Source: three-view drawing plus pictorial views. Frame: mm from the lowest corner of the part. A direction names the side the tool comes from. Round coordinates to 2 decimals unless told otherwise and drop trailing zeros. Loops run counter-clockwise (first coordinate to the right, second up) from the corner with the lowest first, then second, coordinate; pieces in that order, holes last. Notation, with made-up numbers: (57.25, -4) -> (110.25, -4) arc R25 ccw to (110.25, 23) -> close; hole circle Ø1 at (63, 25). An arc over 180 degrees is marked (long way). Answer in a Markdown table with one row per item.
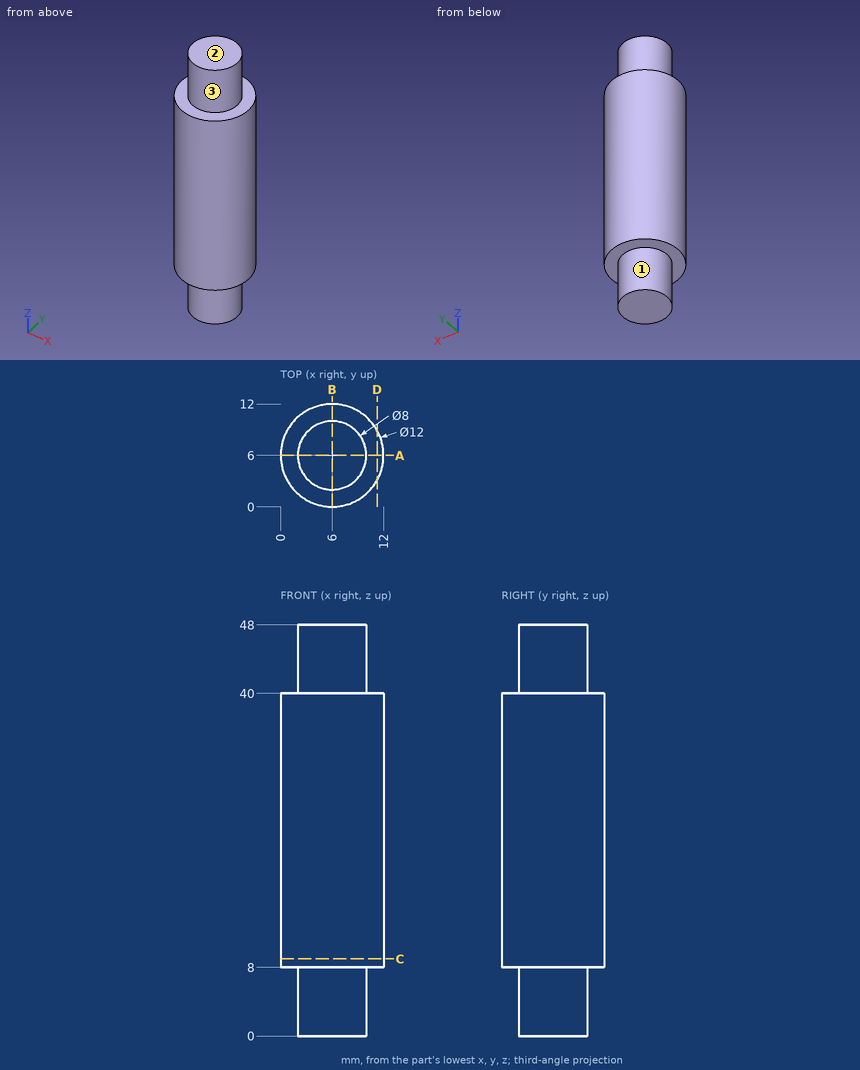
Item 1: Reachability of the marked faces 1, 2 and 3 from +Z, -Z, +X, -X, +Y, -Y: full face, straight path, thin tool, end or side. Return the list, or none.
Answer:
| item | result |
|---|---|
| face 1 | -Z |
| face 2 | +Z, +X, -X, +Y, -Y |
| face 3 | +Z |
Item 2: Cut plane D-D (x = 11.25). Output: boundary loops of the cut face in (y, z).
Answer:
| item | result |
|---|---|
| outline | (3.1, 8) -> (8.9, 8) -> (8.9, 40) -> (3.1, 40) -> close |
Item 3: Cut plane A-A (y = 6). Output: boundary loops of the cut face in (x, z), then the cut area to 3 significant figures.
Answer:
| item | result |
|---|---|
| outline | (0, 8) -> (2, 8) -> (2, 0) -> (10, 0) -> (10, 8) -> (12, 8) -> (12, 40) -> (10, 40) -> (10, 48) -> (2, 48) -> (2, 40) -> (0, 40) -> close |
| area | 512 mm² |
Item 4: Line query: probe 1 along Z at (x, y) = (9.5, 1.25); probe 2 along X at (y, z) = (6.75, 30); probe 3 along Y at (x, z) = (10, 36). Output: solid intervals per line, ascending. Write a range as [from, to].
Answer:
| item | result |
|---|---|
| probe 1 | z = [8, 40] |
| probe 2 | x = [0.05, 11.95] |
| probe 3 | y = [1.53, 10.47] |
Item 5: Cut plane C-C (z = 9). Output: boundary loops of the cut face in (x, y), then the cut area to 3 significant figures.
Answer:
| item | result |
|---|---|
| outline | circle Ø12 at (6, 6) |
| area | 113 mm² |
Item 6: Pin query (flat end, axial travel): pin 1 Ø6 at (x, y) = (6.5, 5.5) entering from -Z; pin 2 Ø1 at (x, z) = (8.5, 8.5) entering from +Y; pin 3 Ø1.5 at (y, z) = (5.5, 42.5) entering from -X; pin 4 Ø1.5 at (x, z) = (3.5, 37) entering from -Y. Return the tip coordinate at first contact, or that it passes through.
Answer:
| item | result |
|---|---|
| pin 1 | stops at z = 0 |
| pin 2 | stops at y = 11.66 |
| pin 3 | stops at x = 2 |
| pin 4 | stops at y = 0.26 |
